Check sheet for the modelled part. Datum: model origin and axes. Units: mm. Face numbers are marked on the shaded views. A direction names the side the tool comes from. Give positions to 0.01 mm unless a question says otherwise; leave off trailing zeros. Loops run counter-clockwise (first coordinate to the right, second up) from the corner with the lowest first, then second, coordinate; pieces in that order, holes last. Notation, with made-up numbers: (-32, 48.5) - (-23, 48.5) arc R22 ccw to (-23, 83.5) - close; hole circle Ø11 at (3.25, -17). An arc over 180 degrees is marked (long way). Use CSV: the item, a comma, the result in double quotes.
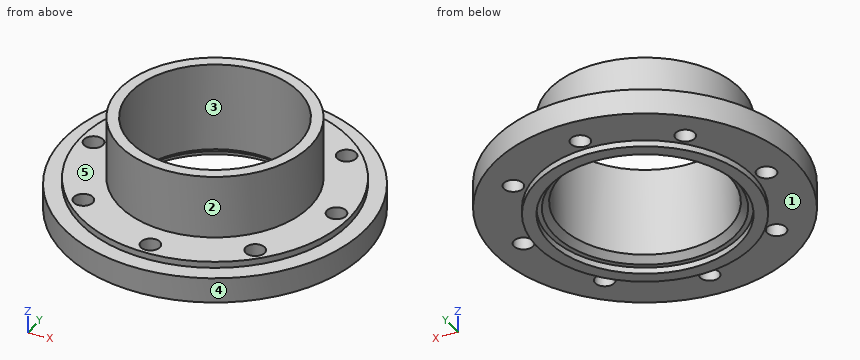
from build123d import *

# Parameters (mm, degrees)
SKETCH_1_R          = 47.5
EXTRUDE_1_DEPTH     = 10
SKETCH_2_R          = 30
EXTRUDE_2_DEPTH     = 20
SKETCH_3_R          = 26.5
CUT_EXTRUDE_1_DEPTH = 40
EXTRUDE_START       = 2
SKETCH_4_R          = 34
SKETCH_4_R_2        = 30
EXTRUDE_3_DEPTH     = 2
CUT_EXTRUDE_START   = -2
SKETCH_5_R          = 47.5
SKETCH_5_R_2        = 42.25
CUT_EXTRUDE_2_DEPTH = 2
SKETCH_6_R          = 3
CUT_EXTRUDE_3_DEPTH = 10
CHAMFER_1_SIZE      = 2


with BuildPart() as part:
    # 草图1 → 拉伸1 (new body)
    with BuildSketch(Plane.XY):
        Circle(SKETCH_1_R)
    extrude(amount=EXTRUDE_1_DEPTH)

    # 草图2 → 拉伸2 (add)
    with BuildSketch(Plane.XY.offset(10)):
        Circle(SKETCH_2_R)
    extrude(amount=EXTRUDE_2_DEPTH)

    # 草图3 → 切除-拉伸1 (cut)
    with BuildSketch(Plane.XY.offset(30)):
        Circle(SKETCH_3_R)
    extrude(amount=-CUT_EXTRUDE_1_DEPTH, mode=Mode.SUBTRACT)

    # 草图4 → 拉伸3 (add)
    with BuildSketch(Plane(origin=(0, 0, 0), x_dir=(-1, 0, 0), z_dir=(0, 0, -1)).offset(EXTRUDE_START)):
        with Locations(Location((0, 0, 0), (0, 0, 180))):
            Circle(SKETCH_4_R)
        with Locations(Location((0, 0, 0), (0, 0, 180))):
            Circle(SKETCH_4_R_2, mode=Mode.SUBTRACT)
    extrude(amount=-EXTRUDE_3_DEPTH)

    # 草图5 → 切除-拉伸2 (cut)
    with BuildSketch(Plane.XY.offset(10).offset(CUT_EXTRUDE_START)):
        Circle(SKETCH_5_R)
        Circle(SKETCH_5_R_2, mode=Mode.SUBTRACT)
    extrude(amount=CUT_EXTRUDE_2_DEPTH, mode=Mode.SUBTRACT)

    # 草图6 → 切除-拉伸3 (cut)
    with BuildSketch(Plane.XY.offset(10)):
        with Locations((26.870057685, 26.870057685)):
            Circle(SKETCH_6_R)
        with Locations((0, 38)):
            Circle(SKETCH_6_R)
        with Locations((38, 0)):
            Circle(SKETCH_6_R)
        with Locations((26.870057685, -26.870057685)):
            Circle(SKETCH_6_R)
        with Locations((0, -38)):
            Circle(SKETCH_6_R)
        with Locations((-26.870057685, -26.870057685)):
            Circle(SKETCH_6_R)
        with Locations((-38, 0)):
            Circle(SKETCH_6_R)
        with Locations((-26.870057685, 26.870057685)):
            Circle(SKETCH_6_R)
    extrude(amount=-CUT_EXTRUDE_3_DEPTH, mode=Mode.SUBTRACT)

    # 倒角1
    chamfer_1_edges = [part.edges().sort_by_distance(p)[0] for p in [
        (-26.5, 0, 0),
    ]]
    chamfer(chamfer_1_edges, length=CHAMFER_1_SIZE)


solid = part.part
1. Scan lines: line 1 along Y through (x, z) = (0, 7.25); line 2 along Y through (x, z) = (-38, 4.25); line 3 along Y through (x, z) = (0, 21). Record each from-to range of solid material in increasing order.
Completed:
line 1,"y = -47.5 to -41, -35 to -26.5, 26.5 to 35, 41 to 47.5"
line 2,"y = -28.5 to -3, 3 to 28.5"
line 3,"y = -30 to -26.5, 26.5 to 30"
2. Release check for a two-part mould opening along Y. For the marked faces 3, 4 and 5 record: released by +Y, released by -Y, zero draft, split by the parting line, or undercut.
Completed:
face 3,"undercut"
face 4,"split by the parting line"
face 5,"zero draft"
3. Go/stop test with flat-tipped pins: pin 1 Ø6 at (x, z) = (9, 16.5) entering from -Y; pin 2 Ø10 at (y, z) = (-22.5, 10) entering from +X; pin 3 Ø6 at (x, z) = (-7, 22.5) entering from +Y. Record where each tip stops, or that it passes through.
Completed:
pin 1,"stops at y = -29.39"
pin 2,"stops at x = 43.99"
pin 3,"stops at y = 29.73"
4. Sectioned sample at A-A, the plane y = 0. State how many separate pieces and enclosed holes the cut face has, and give its area (3 significant figures).
Completed:
separate pieces,"4"
enclosed holes,"0"
area,"431 mm²"
5. Set-up check for the marked faces 1 and 2: record each of +Z, -Z, +X, -X, +Y, -Y from which the full face is reachable in a straight line by a thin tool's end or side.
Completed:
face 1,"-Z"
face 2,"+Z"
6. Sectioned sample at C-C, the plane z = 23. Record the boundary of the cut face in (x, y).
Completed:
outline,"circle Ø60 at (0, 0); hole circle Ø53 at (0, 0)"
7. Sectioned sample at D-D, the plane x = -38. Record the boundary of the cut face in (y, z).
Completed:
outline,"(-28.5, 0) - (-3, 0) - (-3, 10) - (-18.47, 10) - (-18.47, 8) - (-28.5, 8) - close; (3, 0) - (28.5, 0) - (28.5, 8) - (18.47, 8) - (18.47, 10) - (3, 10) - close"
